Could you check a few things on this model? Use its own coordinates, in mm. A direction names the side the tool comes from. Give positions to 0.01 mm unless a question says otherwise; leave off trailing zeros. Loops run counter-clockwise (first coordinate to the right, second up) from the corner with the lowest first, then second, coordinate; pieces in that order, holes last. Notation, with made-up numbers: M 26,-38.5 L 39,-38.5 A9 ccw 39,-24.5 Z; hole C 43.5,-21 d6. An arc over 180 degrees is marked long. Answer in a Markdown table with one row per item. Add a question column.
1. Thinking about a two-plate mould opening in Y: for faces 1 (the cylindrical face through (2.43, 2.23, 1.57)), 2 (the cylindrical face through (-30.495, 0.244, 1.191)), 3 (the flat face through (-10, -17.462, 3)), 4 (the flat face through (0, 17.462, 2)), which applies, released by +Y, released by -Y, zero draft, split by the parting line, or undercut?
2. If we section it at A-A on x = 0: List the corners of the cut face in (y, z) for me (1 decimal), then the cut area to 3 significant figures.
3. Which directions (+Z, -Z, +X, -X, +Y, -Y) give clear straight access to the entire face, cutting with the end or side of a thin tool? Please do faces 5 (the flat face through (2, -4, 3.175)), 6 (the flat face through (-30.18, 0.24, 25.6)).
4. If we section it at D-D on x = -24.5: List the corners of the cut face in (y, z) for me (1 decimal), then the cut area to 3 significant figures.
5. If we section it at C-C on y = 7.5: List the corners of the cut face in (x, z) for me (3 decimals).
6. I need wall thicknesses on line 1 along Z through (x, y) = (4.5, -15) (3 decimals); line 2 along Y through (x, z) = (0, 0.8); line 3 along X through (y, z) = (8.5, 14) (3 decimals). Which ranges of each line are inside material? Lowest first, please. Write a range as from..to.
7. I'm going to push flat-ended pins straight in: pin 1 Ø1 at (x, y) = (5.5, -13.5) entering from +Z (3 decimals); pin 2 Ø5 at (y, z) = (12, 12.5) entering from +X (3 decimals); pin 3 Ø6 at (y, z) = (-3, 35) entering from -X. Where does each tip first touch, or does it pass through?
8. If we section it at B-B on y = 0: List the corners of the cut face in (x, z) for me (3 decimals).
```python
from build123d import *

# Parameters (mm, degrees)
SKETCH2_W                    = 57.15
SKETCH2_H                    = 34.925
BASE_FLANGE1_DEPTH           = 3.175
M6_CLEARANCE_HOLE1_D         = 6.6
EDGE_FLANGE2_STRIP_W         = 14.7
EDGE_FLANGE2_STRIP_H         = 3.175
EDGE_FLANGE2_STRIP_CUT_DEPTH = 34.925
EDGE_FLANGE2_DEPTH           = 34.925
CUT_EXTRUDE2_DEPTH           = 79.817416579
SKETCH21_W                   = 3.175
SKETCH21_H                   = 34.925
BOSS_EXTRUDE1_DEPTH          = 3.175


# Sheet-metal steps are written as plain solids
with BuildPart() as part:
    # Sketch2 → Base-Flange1 (new body)
    with BuildSketch(Plane.XY):
        Rectangle(SKETCH2_W, SKETCH2_H)
    extrude(amount=BASE_FLANGE1_DEPTH)

    # M6 Clearance Hole1 (through all)
    with Locations(Plane.XY.offset(3.175)):
        with Locations((0, 0)):
            Hole(M6_CLEARANCE_HOLE1_D / 2)

    # Edge-Flange2 strip (across the edge) → Edge-Flange2 strip cut (cut)
    with BuildSketch(Plane(origin=(-28.575, 17.4625, 3.175), x_dir=(1, 0, 0), z_dir=(0, -1, 0))):
        with Locations((-6.35, -1.5875)):
            Rectangle(EDGE_FLANGE2_STRIP_W, EDGE_FLANGE2_STRIP_H)
    extrude(amount=EDGE_FLANGE2_STRIP_CUT_DEPTH, mode=Mode.SUBTRACT)

    # Edge-Flange2 section (across the edge) → Edge-Flange2 (add)
    with BuildSketch(Plane(origin=(-28.575, 17.4625, 3.175), x_dir=(1, 0, 0), z_dir=(0, -1, 0))):
        with BuildLine():
            Line((-3.175, 1), (-3.175, 44.45))
            Line((-3.175, 44.45), (0, 44.45))
            Line((0, 44.45), (0, 1))
            ThreePointArc((0, 1), (0.292893219, 0.292893219), (1, 0))
            Line((1, 0), (1, -3.175))
            ThreePointArc((1, -3.175), (-1.952170811, -1.952170811), (-3.175, 1))
        make_face()
    extrude(amount=EDGE_FLANGE2_DEPTH)

    # Sketch20 → Cut-Extrude2 (cut, through all)
    with BuildSketch(Plane.ZY.offset(31.75)):
        Polygon((4.175, 17.4625), (47.625, -17.4625), (47.625, 17.4625), align=None)
    extrude(amount=-CUT_EXTRUDE2_DEPTH, mode=Mode.SUBTRACT)

    # Sketch21 → Boss-Extrude1 (add)
    with BuildSketch(Plane(origin=(28.575, 0, 0), x_dir=(0, 0, -1), z_dir=(1, 0, 0))):
        with Locations((-1.5875, 0)):
            Rectangle(SKETCH21_W, SKETCH21_H)
    extrude(amount=BOSS_EXTRUDE1_DEPTH)


solid = part.part
```
Results:
| question | item | result |
|---|---|---|
| 1 | face 1 | undercut |
| 1 | face 2 | zero draft |
| 1 | face 3 | released by -Y |
| 1 | face 4 | released by +Y |
| 2 | outline | M -17.5,0 L -3.3,0 L -3.3,3.2 L -17.5,3.2 Z; M 3.3,0 L 17.5,0 L 17.5,3.2 L 3.3,3.2 Z |
| 2 | area | 89.9 mm2 |
| 3 | face 5 | +Z, +X, +Y, -Y |
| 3 | face 6 | +Z, +X, -X, +Y |
| 4 | outline | M -17.5,0 L 17.5,0 L 17.5,3.2 L -17.5,3.2 Z |
| 4 | area | 111 mm2 |
| 5 | outline | M -31.75,4.175 A4.175 ccw -27.575,0 L 31.75,0 L 31.75,3.175 L -27.575,3.175 A1 cw -28.575,4.175 L -28.575,16.569 L -31.75,16.569 Z |
| 6 | line 1 | 0..3.175 |
| 6 | line 2 | -17.46..-3.3, 3.3..17.46 |
| 6 | line 3 | -31.75..-28.575 |
| 7 | pin 1 | z = 3.175 |
| 7 | pin 2 | x = -28.575 |
| 7 | pin 3 | through |
| 8 | outline | M -31.75,4.175 A4.175 ccw -27.575,0 L -3.3,0 L -3.3,3.175 L -27.575,3.175 A1 cw -28.575,4.175 L -28.575,25.9 L -31.75,25.9 Z; M 3.3,0 L 31.75,0 L 31.75,3.175 L 3.3,3.175 Z |
